For this review, take the finished solid that the model builds, in its own axes (mm). A direction names the side the tool comes from. Give positions to 0.01 mm unless a question says otherwise; leave off trailing zeros. Loops run counter-clockwise (first coordinate to the right, second up) from the corner with the lowest first, then second, coordinate; pieces in that order, holes last.
```python
from build123d import *

# Parameters (mm, degrees)
SKETCH1_W           = 300
SKETCH1_H           = 200
BOSS_EXTRUDE1_DEPTH = 37.5
SHELL1_T            = -5
FILLET1_R           = 10
SKETCH2_R           = 7.5
CUT_EXTRUDE1_DEPTH  = 5
SKETCH3_R           = 7.5
CUT_EXTRUDE2_DEPTH  = 5
SKETCH4_R           = 10
CUT_EXTRUDE3_DEPTH  = 5
BOSS_EXTRUDE2_START = 15
SKETCH5_R           = 10
SKETCH5_R_2         = 7.5
BOSS_EXTRUDE2_DEPTH = 15
SKETCH6_R           = 10
SKETCH6_R_2         = 7.5
BOSS_EXTRUDE3_DEPTH = 15
SKETCH7_R           = 12.5
SKETCH7_R_2         = 10
BOSS_EXTRUDE4_DEPTH = 15


with BuildPart() as part:
    # Sketch1 → Boss-Extrude1 (new, symmetric)
    with BuildSketch(Plane(origin=(0, 0, 0), x_dir=(1, 0, 0), z_dir=(0, 1, 0))):
        Rectangle(SKETCH1_W, SKETCH1_H)
    extrude(amount=BOSS_EXTRUDE1_DEPTH, both=True)

    # Shell1
    shell1_openings = [part.faces().sort_by_distance(p)[0] for p in [
        (0, 37.5, 0),
    ]]
    offset(amount=SHELL1_T, openings=shell1_openings, kind=Kind.INTERSECTION)

    # Fillet1
    fillet1_edges = [part.edges().sort_by_distance(p)[0] for p in [
        (-145, -32.5, 0),
        (-145, 2.5, -95),
        (0, -32.5, 95),
        (-145, 2.5, 95),
        (145, -32.5, 0),
        (145, 2.5, 95),
        (0, -32.5, -95),
        (145, 2.5, -95),
    ]]
    fillet(fillet1_edges, radius=FILLET1_R)

    # Sketch2 → Cut-Extrude1 (cut)
    with BuildSketch(Plane(origin=(150, 0, 0), x_dir=(0, 0, -1), z_dir=(1, 0, 0))):
        with Locations((75, 0)):
            Circle(SKETCH2_R)
        with Locations((25, 0)):
            Circle(SKETCH2_R)
        with Locations((-75, 0)):
            Circle(SKETCH2_R)
    extrude(amount=-CUT_EXTRUDE1_DEPTH, mode=Mode.SUBTRACT)

    # Sketch3 → Cut-Extrude2 (cut)
    with BuildSketch(Plane(origin=(-145, 0, 0), x_dir=(0, 0, -1), z_dir=(1, 0, 0))):
        with Locations((-50, 0)):
            Circle(SKETCH3_R)
    extrude(amount=-CUT_EXTRUDE2_DEPTH, mode=Mode.SUBTRACT)

    # Sketch4 → Cut-Extrude3 (cut)
    with BuildSketch(Plane.XY.offset(-95)):
        Circle(SKETCH4_R)
    extrude(amount=-CUT_EXTRUDE3_DEPTH, mode=Mode.SUBTRACT)

    # Sketch5 → Boss-Extrude2 (add)
    # profile 1 of 3: a face of its own
    with BuildSketch(Plane(origin=(150, 0, 0), x_dir=(0, 0, -1), z_dir=(1, 0, 0)).offset(BOSS_EXTRUDE2_START)):
        with Locations(Location((-75, 0, 0), (0, 0, 180))):
            Circle(SKETCH5_R)
        with Locations((-75, 0)):
            Circle(SKETCH5_R_2, mode=Mode.SUBTRACT)
    # profile 2 of 3: a face of its own
    with BuildSketch(Plane(origin=(150, 0, 0), x_dir=(0, 0, -1), z_dir=(1, 0, 0)).offset(BOSS_EXTRUDE2_START)):
        with Locations(Location((25, 0, 0), (0, 0, 180))):
            Circle(SKETCH5_R)
        with Locations((25, 0)):
            Circle(SKETCH5_R_2, mode=Mode.SUBTRACT)
    # profile 3 of 3: a face of its own
    with BuildSketch(Plane(origin=(150, 0, 0), x_dir=(0, 0, -1), z_dir=(1, 0, 0)).offset(BOSS_EXTRUDE2_START)):
        with Locations(Location((75, 0, 0), (0, 0, 180))):
            Circle(SKETCH5_R)
        with Locations((75, 0)):
            Circle(SKETCH5_R_2, mode=Mode.SUBTRACT)
    extrude(amount=-BOSS_EXTRUDE2_DEPTH)

    # Sketch6 → Boss-Extrude3 (add)
    with BuildSketch(Plane.ZY.offset(150)):
        with Locations(Location((50, 0, 0), (0, 0, 180))):
            Circle(SKETCH6_R)
        with Locations(Location((50, 0, 0), (0, 0, 180))):
            Circle(SKETCH6_R_2, mode=Mode.SUBTRACT)
    extrude(amount=BOSS_EXTRUDE3_DEPTH)

    # Sketch7 → Boss-Extrude4 (add)
    with BuildSketch(Plane(origin=(0, 0, -100), x_dir=(-1, 0, 0), z_dir=(0, 0, -1))):
        with Locations(Location((0, 0, 0), (0, 0, 180))):
            Circle(SKETCH7_R)
        with Locations(Location((0, 0, 0), (0, 0, 180))):
            Circle(SKETCH7_R_2, mode=Mode.SUBTRACT)
    extrude(amount=BOSS_EXTRUDE4_DEPTH)


solid = part.part
```
Item 1: For L1, parallel to X at y = 30, z = -68.5; L2, parallel to Y at x = 159.5, z = 75; L3, parallel to Z at x = -41, y = 0.5, list the stretches that pass through material, from the lowest coordinate up.
Answer:
L1: x = -150 to -145, 145 to 150
L2: y = -10 to -7.5, 7.5 to 10
L3: z = -100 to -95, 95 to 100
Item 2: Take a section at B-B on z = -75. Give the boundary of the cut face in (x, y).
Answer:
outline: (-150, -37.5) - (150, -37.5) - (150, -10) - (165, -10) - (165, -7.5) - (145, -7.5) - (145, -22.5) arc R10 cw to (135, -32.5) - (-135, -32.5) arc R10 cw to (-145, -22.5) - (-145, 37.5) - (-150, 37.5) - close; (145, 7.5) - (165, 7.5) - (165, 10) - (150, 10) - (150, 37.5) - (145, 37.5) - close
Item 3: Take a section at D-D on x = -60.5. Give the boundary of the cut face in (y, z).
Answer:
outline: (-37.5, -100) - (37.5, -100) - (37.5, -95) - (-22.5, -95) arc R10 cw to (-32.5, -85) - (-32.5, 85) arc R10 cw to (-22.5, 95) - (37.5, 95) - (37.5, 100) - (-37.5, 100) - close
Item 4: Take a section at A-A on x = 0. Give the boundary of the cut face in (y, z), and give its area (3 significant figures).
Answer:
outline: (-37.5, -100) - (-12.5, -100) - (-12.5, -115) - (-10, -115) - (-10, -95) - (-22.5, -95) arc R10 cw to (-32.5, -85) - (-32.5, 85) arc R10 cw to (-22.5, 95) - (37.5, 95) - (37.5, 100) - (-37.5, 100) - close; (10, -115) - (12.5, -115) - (12.5, -100) - (37.5, -100) - (37.5, -95) - (10, -95) - close
area: 1,720 mm2
Item 5: The part is to be moulded in two halves that separate along Z. For faces 1 (the cylindrical face through (-157, 0, 60)), 2 (the cylindrical face through (-1.89, -29.49, -92.15)), 3 (the flat face through (165, -7, -71)), say which applies: released by +Z, released by -Z, zero draft, split by the parting line, or undercut.
Answer:
face 1: split by the parting line
face 2: undercut
face 3: zero draft
Item 6: Clearance check with flat-ended pins moving along their axes: pin 1 Ø12 at (y, z) = (0, 75) entering from +X; pin 2 Ø8 at (x, y) = (45, 28.5) entering from -Z; pin 3 Ø6 at (x, z) = (93.5, 19) entering from +Y. State where each tip first meets the part, or that it passes through.
Answer:
pin 1: stops at x = -145
pin 2: stops at z = -100
pin 3: stops at y = -32.5
Item 7: Tool access review of faces 4 (the cylindrical face through (142.15, 7.08, 91.99)), 5 (the flat face through (150, 1, 1)), 6 (the cylindrical face through (11.923, -3.755, -107.395)), 7 (the flat face through (-0.1, -10.2, -115)): name each direction out of +Z, -Z, +X, -X, +Y, -Y from which nothing blocks a thin tool from reaching the whole face with its end or side.
Answer:
face 4: +Y
face 5: +X
face 6: -Z
face 7: -Z, +X, -X, +Y, -Y
Item 8: Take a section at C-C on y = 29. Give the boundary of the cut face in (x, z), and give its area (3 significant figures).
Answer:
outline: (-150, -100) - (150, -100) - (150, 100) - (-150, 100) - close; hole (-145, -85) arc R10 ccw to (-135, -95) - (135, -95) arc R10 ccw to (145, -85) - (145, 85) arc R10 ccw to (135, 95) - (-135, 95) arc R10 ccw to (-145, 85) - close
area: 4,990 mm2
